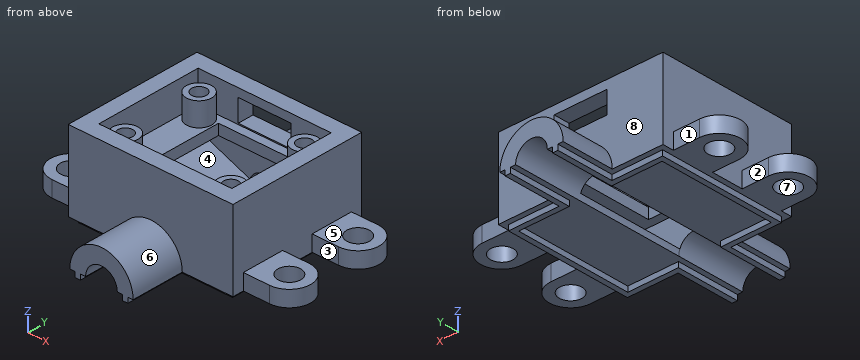
from build123d import *

# Parameters (mm, degrees)
SKETCH1_W            = 31.2
SKETCH1_H            = 26.2
BOSS_EXTRUDE1_DEPTH  = 15
SHELL2_T             = -3
BOSS_EXTRUDE2_DEPTH  = 10
CUT_EXTRUDE2_DEPTH   = 43.175822458
SKETCH8_R            = 2.15
BOSS_EXTRUDE5_DEPTH  = 3
BOSS_EXTRUDE4_DEPTH  = 1
SKETCH14_W           = 25.2
SKETCH14_H           = 20.2
CUT_EXTRUDE5_DEPTH   = 37.163102743
BOSS_EXTRUDE8_REACH  = 45.959
BOSS_EXTRUDE9_START  = -8
SKETCH15_W           = 31.2
SKETCH15_H           = 26.2
SKETCH15_W_2         = 14.5
SKETCH15_H_2         = 17
BOSS_EXTRUDE9_DEPTH  = 2
SKETCH16_R           = 2.4
SKETCH16_R_2         = 1.4
BOSS_EXTRUDE10_DEPTH = 4.41
CUT_EXTRUDE6_REACH   = 48.267
SKETCH5_W            = 10
SKETCH5_H            = 4.18


with BuildPart() as part:
    # Sketch1 → Boss-Extrude1 (new body)
    with BuildSketch(Plane.XY):
        Rectangle(SKETCH1_W, SKETCH1_H)
    extrude(amount=BOSS_EXTRUDE1_DEPTH)

    # Shell2
    shell2_openings = [part.faces().sort_by_distance(p)[0] for p in [
        (0, 0, 0),
    ]]
    offset(amount=SHELL2_T, openings=shell2_openings, kind=Kind.INTERSECTION)

    # Sketch3 → Boss-Extrude2 (add)
    with BuildSketch(Plane(origin=(0, 13.1, 0), x_dir=(1, 0, 0), z_dir=(0, 1, 0))):
        with BuildLine():
            Line((-6, 0), (-3, 0))
            ThreePointArc((-3, 0), (0, -3), (3, 0))
            Line((3, 0), (6, 0))
            ThreePointArc((6, 0), (0, -6), (-6, 0))
        make_face()
    boss_extrude2 = extrude(amount=BOSS_EXTRUDE2_DEPTH)

    # Mirror1: Boss-Extrude2 across plane
    add(boss_extrude2.mirror(Plane.ZX))

    # Sketch4 → Cut-Extrude2 (cut, through all)
    with BuildSketch(Plane(origin=(0, 13.1, 0), x_dir=(1, 0, 0), z_dir=(0, 1, 0))):
        with BuildLine():
            Line((-3, 0), (3, 0))
            ThreePointArc((3, 0), (0, -3), (-3, 0))
        make_face()
    extrude(amount=-CUT_EXTRUDE2_DEPTH, mode=Mode.SUBTRACT)

    # Sketch8 → Boss-Extrude5 (add)
    # profile 1 of 2: a face of its own
    with BuildSketch(Plane(origin=(0, 0, 0), x_dir=(-1, 0, 0), z_dir=(0, 0, -1))):
        with BuildLine():
            Line((-15.6, 3), (-15.6, 11))
            Line((-15.6, 11), (-20.6, 11))
            ThreePointArc((-20.6, 11), (-24.6, 7), (-20.6, 3))
            Line((-20.6, 3), (-15.6, 3))
        make_face()
        with Locations((-20.6, 7)):
            Circle(SKETCH8_R, mode=Mode.SUBTRACT)
    # profile 2 of 2: a face of its own
    with BuildSketch(Plane(origin=(0, 0, 0), x_dir=(-1, 0, 0), z_dir=(0, 0, -1))):
        with BuildLine():
            Line((-15.6, -11), (-15.6, -3))
            Line((-15.6, -3), (-20.6, -3))
            ThreePointArc((-20.6, -3), (-24.6, -7), (-20.6, -11))
            Line((-20.6, -11), (-15.6, -11))
        make_face()
        with Locations((-20.6, -7)):
            Circle(SKETCH8_R, mode=Mode.SUBTRACT)
    boss_extrude5 = extrude(amount=-BOSS_EXTRUDE5_DEPTH)

    # Mirror3: Boss-Extrude5 across plane
    add(boss_extrude5.mirror(Plane(origin=(0, 0, 0), x_dir=(0, 0, 1), z_dir=(1, 0, 0))))

    # Sketch7 → Boss-Extrude4 (add)
    with BuildSketch(Plane(origin=(0, 0, 0), x_dir=(-1, 0, 0), z_dir=(0, 0, -1))):
        Polygon((-4, -23.1), (-4, -11.1), (-13.6, -11.1), (-13.6, 11.1), (-4, 11.1), (-4, 23.1), (-5, 23.1), (-5, 12.1), (-14.6, 12.1), (-14.6, -12.1), (-5, -12.1), (-5, -23.1), align=None)
    boss_extrude4 = extrude(amount=BOSS_EXTRUDE4_DEPTH)

    # Mirror2: Boss-Extrude4 across plane
    add(boss_extrude4.mirror(Plane(origin=(0, 0, 0), x_dir=(0, 0, 1), z_dir=(1, 0, 0))))

    # Sketch14 → Cut-Extrude5 (cut, through all)
    with BuildSketch(Plane(origin=(0, 0, 12), x_dir=(-1, 0, 0), z_dir=(0, 0, -1))):
        Rectangle(SKETCH14_W, SKETCH14_H)
    extrude(amount=-CUT_EXTRUDE5_DEPTH, mode=Mode.SUBTRACT)

    # Sketch11 → Boss-Extrude8 (add, up to next)
    with BuildSketch(Plane(origin=(0, -10.1, 0), x_dir=(1, 0, 0), z_dir=(0, 1, 0)), mode=Mode.PRIVATE) as boss_extrude8_sk1:
        with BuildLine():
            Line((3, 0), (12.6, 0))
            Line((12.6, 0), (12.6, -5.002969955))
            Line((12.6, -5.002969955), (2.801311304, -1.073617705))
            ThreePointArc((2.801311304, -1.073617705), (2.949909652, -0.545924027), (3, 0))
        make_face()
    boss_extrude8_tool1 = extrude(boss_extrude8_sk1.sketch, amount=BOSS_EXTRUDE8_REACH, mode=Mode.PRIVATE) - part.part
    # Sketch11 → Boss-Extrude8 (add, up to next)
    with BuildSketch(Plane(origin=(0, -10.1, 0), x_dir=(1, 0, 0), z_dir=(0, 1, 0)), mode=Mode.PRIVATE) as boss_extrude8_sk2:
        with BuildLine():
            Line((-12.6, -5.002969955), (-2.801311304, -1.073617705))
            ThreePointArc((-2.801311304, -1.073617705), (-2.949909652, -0.545924027), (-3, 0))
            Line((-3, 0), (-12.6, 0))
            Line((-12.6, 0), (-12.6, -5.002969955))
        make_face()
    boss_extrude8_tool2 = extrude(boss_extrude8_sk2.sketch, amount=BOSS_EXTRUDE8_REACH, mode=Mode.PRIVATE) - part.part
    add(boss_extrude8_tool1.solids().sort_by_distance((8.785084, -10.1, 1.737296))[0])
    add(boss_extrude8_tool2.solids().sort_by_distance((-8.785084, -10.1, 1.737296))[0])

    # Sketch15 → Boss-Extrude9 (add)
    with BuildSketch(Plane.XY.offset(15).offset(BOSS_EXTRUDE9_START)):
        Rectangle(SKETCH15_W, SKETCH15_H)
        Rectangle(SKETCH15_W_2, SKETCH15_H_2, mode=Mode.SUBTRACT)
    extrude(amount=BOSS_EXTRUDE9_DEPTH)

    # Sketch16 → Boss-Extrude10 (add)
    # profile 1 of 4: a face of its own
    with BuildSketch(Plane.XY.offset(9)):
        with Locations((-10, 7.5)):
            Circle(SKETCH16_R)
        with Locations((-10, 7.5)):
            Circle(SKETCH16_R_2, mode=Mode.SUBTRACT)
    # profile 2 of 4: a face of its own
    with BuildSketch(Plane.XY.offset(9)):
        with Locations((10, 7.5)):
            Circle(SKETCH16_R)
        with Locations((10, 7.5)):
            Circle(SKETCH16_R_2, mode=Mode.SUBTRACT)
    # profile 3 of 4: a face of its own
    with BuildSketch(Plane.XY.offset(9)):
        with Locations((-10, -7.5)):
            Circle(SKETCH16_R)
        with Locations((-10, -7.5)):
            Circle(SKETCH16_R_2, mode=Mode.SUBTRACT)
    # profile 4 of 4: a face of its own
    with BuildSketch(Plane.XY.offset(9)):
        with Locations((10, -7.5)):
            Circle(SKETCH16_R)
        with Locations((10, -7.5)):
            Circle(SKETCH16_R_2, mode=Mode.SUBTRACT)
    extrude(amount=BOSS_EXTRUDE10_DEPTH)

    # Sketch5 → Cut-Extrude6 (cut, up to next)
    with BuildSketch(Plane(origin=(0, 13.1, 0), x_dir=(1, 0, 0), z_dir=(0, 1, 0)), mode=Mode.PRIVATE) as cut_extrude6_sk1:
        with Locations((0, -11.31)):
            Rectangle(SKETCH5_W, SKETCH5_H)
    cut_extrude6_tool1 = extrude(cut_extrude6_sk1.sketch, amount=-CUT_EXTRUDE6_REACH, mode=Mode.PRIVATE) & part.part
    add(cut_extrude6_tool1.solids().sort_by_distance((0, 13.1, 11.31))[0], mode=Mode.SUBTRACT)


solid = part.part
The model under review builds one solid part; all positions refer to its coordinate system, in mm. Face numbers are marked on the shaded views. A direction names the side the tool comes from. Coordinates: 2 decimals unless noted, no trailing zeros. Write each loop counter-clockwise with the first axis right and the second up, starting at its lowest first coordinate (ties: lowest second). Pieces come first, ordered by that corner, then holes. Notation, with made-up numbers: M 29.25,6 L 33.25,6 A17 ccw 33.25,10 Z; hole C 23.25,81.5 d6. An arc over 180 degrees is marked long. Put each result on its own line as item: value.
1) For the marked faces 1, 2, 3, 4 and 5, list the 3-axis set-ups (+Z, -Z, +X, -X, +Y, -Y) from which the entire face can be reached by the end or side of a thin tool; tool diameter is ignored.
Computed:
face 1: +Z, -Z, -X, +Y
face 2: +Z, -Z, -X
face 3: +Z, -Z, +X
face 4: none
face 5: +Z, +X, +Y, -Y
2) Clearance check with flat-ended pins moving along their axes: pin 1 Ø3 at (x, z) = (-14.5, 11) entering from +Y; pin 2 Ø1.1 at (y, z) = (0.5, -0.5) entering from -X; pin 3 Ø6.5 at (x, y) = (20.5, 6) entering from +Z. State where each tip first meets the part, or that it passes through.
Computed:
pin 1: stops at y = 13.1
pin 2: stops at x = -15.6
pin 3: stops at z = 3
3) Add section A-A on z = 14.25. Give the boundary of the cut face in (x, y), then the cut area to 3 significant figures.
Computed:
outline: M -15.6,-13.1 L 15.6,-13.1 L 15.6,13.1 L -15.6,13.1 Z; hole M -12.6,-10.1 L 12.6,-10.1 L 12.6,10.1 L -12.6,10.1 Z
area: 308 mm2
4) Wall thickness on probe 1 along Y at (x, z) = (-10, 10.35); probe 2 along Y at (x, z) = (-20.6, 2); probe 3 along X at (y, z) = (-8, 5.5): over which ranges is each line inside the solid? List them lowest first. Write a range as [from, to].
Computed:
probe 1: y = [-13.1, -10.1], [-9.9, -8.9], [-6.1, -5.1], [5.1, 6.1], [8.9, 9.9], [10.1, 13.1]
probe 2: y = [-11, -9.15], [-4.85, -3], [3, 4.85], [9.15, 11]
probe 3: x = [-15.6, -12.6], [12.6, 15.6]
5) Add section D-D on y = 20.5. Give the boundary of the cut face in (x, z), then the cut area to 3 significant figures.
Computed:
outline: M -6,0 L -5,0 L -5,-1 L -4,-1 L -4,0 L -3,0 A3 cw 3,0 L 4,0 L 4,-1 L 5,-1 L 5,0 L 6,0 A6 ccw Z
area: 44.4 mm2
6) Draft analysis for pull direction Y (two halves, no side actions). For the marked faces 6, 7 and 8, state which applies: released by +Y, released by -Y, zero draft, split by the parting line, or undercut.
Computed:
face 6: zero draft
face 7: undercut
face 8: released by +Y
7) Add section B-B on y = -1. Give the boundary of the cut face in (x, z).
Computed:
outline: M -15.6,0 L -14.6,0 L -14.6,-1 L -13.6,-1 L -13.6,0 L -3,0 A3 cw -2.8,1.07 L -12.6,5 L -12.6,7 L -7.25,7 L -7.25,9 L -12.6,9 L -12.6,15 L -15.6,15 Z; M 2.8,1.07 A3 cw 3,0 L 13.6,0 L 13.6,-1 L 14.6,-1 L 14.6,0 L 15.6,0 L 15.6,15 L 12.6,15 L 12.6,9 L 7.25,9 L 7.25,7 L 12.6,7 L 12.6,5 Z
8) Add section C-C on x = -1. Give the boundary of the cut face in (y, z), then the cut area to 3 significant figures.
Computed:
outline: M -23.1,2.83 L -10.1,2.83 L -10.1,7 L -8.5,7 L -8.5,9 L -10.1,9 L -10.1,15 L -13.1,15 L -13.1,5.92 L -23.1,5.92 Z; M 8.5,7 L 10.1,7 L 10.1,2.83 L 23.1,2.83 L 23.1,5.92 L 13.1,5.92 L 13.1,9.22 L 10.1,9.22 L 10.1,9 L 8.5,9 Z; M 10.1,13.4 L 13.1,13.4 L 13.1,15 L 10.1,15 Z
area: 129 mm2
